from build123d import *

# Parameters (mm, degrees)
BOSS_EXTRUDE1_DEPTH = 5.08
SKETCH5_W           = 56.19760994
SKETCH5_H           = 25.4
CUT_EXTRUDE1_DEPTH  = 50.8


with BuildPart() as part:
    # Sketch1 → Boss-Extrude1 (new body)
    with BuildSketch(Plane(origin=(0, 0, 0), x_dir=(1, 0, 0), z_dir=(0, 1, 0))):
        Polygon((-101.738774191, -22.048282475), (-101.738774191, -27.128282475), (-86.298774591, -27.128282475), (-86.298774591, -22.048282475), (-70.858774991, -22.048282475), (-70.858774991, -27.128282475), (-55.418775391, -27.128282475), (-55.418775391, -22.048282475), (-39.978775791, -22.048282475), (-39.978775791, -27.128282475), (-24.538776191, -27.128282475), (-24.538776191, -22.048282475), (-19.458776191, -22.048282475), (-19.458776191, -1.728282475), (-24.614597086, -1.728282475), (-24.614597086, 23.671717525), (-19.458776191, 23.671717525), (-19.458776191, 43.991717525), (-24.614597086, 43.991717525), (-24.614597086, 69.391717525), (-19.458776191, 69.391717525), (-19.458776191, 89.711717525), (-24.538776191, 89.711717525), (-24.538776191, 94.109329465), (-39.978775791, 94.109329465), (-39.978775791, 89.711717525), (-55.418775391, 89.711717525), (-55.418775391, 94.109329465), (-70.858774991, 94.109329465), (-70.858774991, 89.711717525), (-86.298774591, 89.711717525), (-86.298774591, 94.109329465), (-101.738774191, 94.109329465), (-101.738774191, 89.711717525), (-106.818774191, 89.711717525), (-106.818774191, 69.391717525), (-101.132207026, 69.391717525), (-101.132207026, 43.991717525), (-106.818774191, 43.991717525), (-106.818774191, 23.671717525), (-101.132207026, 23.671717525), (-101.132207026, -1.728282475), (-106.818774191, -1.728282475), (-106.818774191, -22.048282475), align=None)
    extrude(amount=BOSS_EXTRUDE1_DEPTH)

    # Sketch5 → Cut-Extrude1 (cut)
    with BuildSketch(Plane(origin=(0, 5.08, 0), x_dir=(1, 0, 0), z_dir=(0, 1, 0))):
        with Locations((-62.873402056, 0.811717525)):
            Rectangle(SKETCH5_W, SKETCH5_H)
    extrude(amount=-CUT_EXTRUDE1_DEPTH, mode=Mode.SUBTRACT)


solid = part.part
Can you work these out from the model? Positions are in its coordinate system, mm. A direction names the side the tool comes from. Give positions to 0.01 mm unless a question says otherwise; leave off trailing zeros. Loops run counter-clockwise (first coordinate to the right, second up) from the corner with the lowest first, then second, coordinate; pieces in that order, holes last. Notation, with made-up numbers: (-40, 52.5) - (11, 52.5) arc R28 cw to (11, 83.5) - close; hole circle Ø11 at (47, 80.5). An arc over 180 degrees is marked (long way). Answer as a JSON object with one key per item and string values.
Q1. Which directions (+Z, -Z, +X, -X, +Y, -Y) give clear straight access to the entire face, cutting with the end or side of a thin tool? Please do faces 1 (the flat face through (-104, 3, 22.048)), 2 (the flat face through (-63, 3, 11.888)), 3 (the flat face through (-24.539, 3, -92)), 4 (the flat face through (-22, 3, -23.672)), 5 (the flat face through (-79, 3, 22.048)).
Geometry says:
{"face 1": "+Z, -X, +Y, -Y", "face 2": "+Y, -Y", "face 3": "-Z, +X, +Y, -Y", "face 4": "+X, +Y, -Y", "face 5": "+Z, +Y, -Y"}
Q2. If I drill on L1, parallel to Z at x = -57, y = 4.25; L2, parallel to Z at x = -77, y = 0.6; L3, parallel to X at y = 3.7, z = 3, over which ranges is the centre line in solid material (lowest first)?
Geometry says:
{"L1": "-94.11 to -13.51, 11.89 to 27.13", "L2": "-89.71 to -13.51, 11.89 to 22.05", "L3": "-106.82 to -90.97, -34.77 to -19.46"}
Q3. Imagine slicing it at C-C on z = -47. Write out the boundary of the cut face in (x, y), plus the area to 3 significant figures.
Geometry says:
{"outline": "(-101.13, 0) - (-24.61, 0) - (-24.61, 5.08) - (-101.13, 5.08) - close", "area": "389 mm²"}
Q4. If we mould it in two halves opening along X, with no side actions, what happens to faces 6 (the flat face through (-104, 3, -69.392)), 7 (the flat face through (-86.299, 3, -92)), 8 (the flat face through (-19.459, 3, -79))? For each: pulls with the +X half, pulls with the -X half, needs draft (parallel to the pull), parting line crosses it, or undercut.
Geometry says:
{"face 6": "needs draft", "face 7": "undercut", "face 8": "pulls with the +X half"}
Q5. Will these pins go through, and if not, where does the flat tip stop? P1, Ø2.5, axis at y = 2.5, z = 24, coming from the +X side; P2, Ø2.5, axis at y = 2.5, z = -15.5, coming from the +X side; P3, Ø1.5, axis at y = 2.5, z = -10.5, coming from the -X side.
Geometry says:
{"P1": "x = -24.54", "P2": "x = -24.61", "P3": "x = -101.13"}
Q6. Imagine slicing it at B-B on x = -62.5. Write out the boundary of the cut face in (y, z), plus the area to 3 significant figures.
Geometry says:
{"outline": "(0, -94.11) - (5.08, -94.11) - (5.08, -13.51) - (0, -13.51) - close; (0, 11.89) - (5.08, 11.89) - (5.08, 27.13) - (0, 27.13) - close", "area": "487 mm²"}
Q7. Imagine slicing it at A-A on z = -6.5. Write out the boundary of the cut face in (x, y), plus the area to 3 significant figures.
Geometry says:
{"outline": "(-101.13, 0) - (-90.97, 0) - (-90.97, 5.08) - (-101.13, 5.08) - close; (-34.77, 0) - (-24.61, 0) - (-24.61, 5.08) - (-34.77, 5.08) - close", "area": "103 mm²"}
